Work out the finished part from the listing and answer in its coordinate system (mm). A direction names the side the tool comes from. Round coordinates to 2 decimals unless told otherwise and drop trailing zeros. Loops run counter-clockwise (first coordinate to the right, second up) from the corner with the lowest first, then second, coordinate; pieces in that order, holes last. Notation, with made-up numbers: M -21.5,54.5 L 25.5,54.5 A3 ccw 25.5,59.5 Z; hole C 14.25,80.5 d7. An arc over 180 degrees is marked long. One line per item, written item: value.
Autodesk Inventor part; units mm, degrees
ref_plane "YZ Plane" through (0, 0, 0) normal (1, 0, 0) x (0, 1, 0)
ref_plane "XZ Plane" through (0, 0, 0) normal (0, 1, 0) x (-1, 0, 0)
ref_plane "XY Plane" through (0, 0, 0) normal (0, 0, 1) x (1, 0, 0)
sketch "Sketch1" plane through (0, 0, 0) normal (0, 0, 1) x (1, 0, 0)
  circle A0 centre (0, 24.7) radius 8.1
  line L0 (0, 24.7) -> (0, 0) construction
  line L1 (0, 0) -> (-20, 0) construction
  line L2 (-20, 5) -> (-9.2, 5)
  line L3 (-9.2, 5) -> (-3.85, 17.5735)
  line L4 (0, 0) -> (20, 0) construction
  line L5 (20, 0) -> (20, 5) construction
  line L6 (20, 5) -> (9.2, 5)
  line L7 (9.2, 5) -> (3.85, 17.5735)
  line L8 (0, 24.7) -> (0, 32.8) construction
  line L9 (-3.85, 17.5735) -> (3.85, 17.5735) construction
  line L10 (-20, 5) -> (-20, 42)
  line L11 (-20, 42) -> (20, 42)
  line L12 (20, 42) -> (20, 5)
  line L13 (-20, 5) -> (-20, 0)
  line L14 (-20, 0) -> (20, 0)
  line L15 (20, 0) -> (20, 5)
  line L16 (-9.2, 5) -> (9.2, 5)
  point P0 (0, 42)
  point P1 (-20, 5)
  dimension "d0" = 16.2
  dimension "d2" = 5
  dimension "d5" = 7.7
  dimension "d91" = 42
  dimension "d102" = 19.7
  dimension "d103" = 18.4
  dimension "d104" = 40
extrude "Extrusion1" add sketch "Sketch1" along normal blind 30 contours A0 L3 L2 L10 L11 L12 L6 L7
extrude "Extrusion2" add sketch "Sketch1" against normal blind 10
sketch "Sketch6" plane through (-20, 42, 30) normal (0, 1, 0) x (1, 0, 0)
  line L0 (0, 40) -> (0, 0)
  line L1 (40, 0) -> (0, 0)
  line L2 (0, 40) -> (40, 0) construction
  line L3 (40, 40) -> (0, 0) construction
  circle A0 centre (35, 5) radius 1.5
  circle A1 centre (5, 5) radius 1.5
  circle A2 centre (5, 35) radius 1.5
  circle A3 centre (35, 35) radius 1.5
  line L4 (35, 35) -> (35, 5) construction
  line L5 (5, 5) -> (35, 5) construction
  line L6 (5, 5) -> (5, 35) construction
  circle A4 centre (20, 20) radius 1.5
  line L7 (40, 40) -> (40, 0)
  line L8 (0, 40) -> (40, 40)
  point P0 (20, 30)
  dimension "d69" = 30
  dimension "d70" = 3
  dimension "d73" = 3
extrude "Extrusion8" cut sketch "Sketch6" against normal blind 5 contours A0 | A1 | A2 | A3
extrude "Extrusion9" cut sketch "Sketch6" against normal through all contours A4
sketch "Sketch8" plane through (20, 5, 30) normal (1, 0, 0) x (0, 0, -1)
  line L0 (0, 0) -> (0, 37)
  line L1 (30, 0) -> (0, 0)
  line L2 (20, 37) -> (20, 15) construction
  line L3 (20, 15) -> (10, 15) construction
  line L4 (20, 15) -> (30, 15) construction
  circle A0 centre (10, 15) radius 1.75
  circle A1 centre (30, 15) radius 1.75
  line L5 (40, 37) -> (0, 37)
  line L6 (30, -5) -> (30, 0)
  line L7 (30, -5) -> (40, -5)
  line L8 (40, 37) -> (40, -5)
  line L9 (20, 33.5954) -> (20, 18.5954) construction
  circle A2 centre (20, 33.5954) radius 1.5
  circle A3 centre (20, 18.5954) radius 1.5
  line L10 (20, 26.0954) -> (0, 26.0954) construction
  point P0 (30, -5)
  point P1 (35, -5)
  dimension "d97" = 3.5
  dimension "d98" = 3.5
  dimension "d105" = 20
  dimension "d106" = 20
  dimension "d107" = 20
  dimension "d108" = 15
  dimension "d109" = 20
  dimension "d110" = 3
extrude "Extrusion12" cut sketch "Sketch8" against normal blind 5 contours A0 | A1 | A2 | A3
mirror "Mirror1" about plane through (0, 0, 0) normal (1, 0, 0) of "Extrusion12"
properties part number "X Axis End_3DPrint"
1) The mould has two halves that part along Y. Classify faces 6 (the face through (-17.54, 25.06, 10.33)), 7 (the face through (17.54, 37.68, 11.19)), 8 (the face through (-15, 37, 25)), 9 (the face through (0, 0, -5)): +Y half, -Y half, draft (parallel to the pull), parting line (faces both ways), or undercut.
Check values:
face 6: undercut
face 7: undercut
face 8: +Y half
face 9: -Y half
2) For faces 1 (the face through (-0.3, 32.794, 14.79)), 2 (the face through (-15, 5, 15)), 3 (the face through (15, 24, 10)), 4 (the face through (-6.56, 11.2, 14.79)), 5 (the face through (-17.535, 18.265, 0.228)), determine the directions among +Z, -Z, +X, -X, +Y, -Y from which every point of the face is accessible in a straight line to the end or side of a thin tool.
Check values:
face 1: +Z
face 2: +Z, +X, -X, -Y
face 3: +X
face 4: +Z, -Y
face 5: -X
3) Find section B-B (y = 8.5). Give the vertices of the cut face in (x, z).
Check values:
outline: M -20,-10 L 20,-10 L 20,30 L 7.71,30 L 7.71,0 L -7.71,0 L -7.71,30 L -20,30 Z
4) Each of these flat-tipped pins is pushed along its axis until it touches: pin 1 (4.5 mm diameter, centred on y = 20, z = 0, fed in from -X); pin 2 (2 mm diameter, centred on y = 20, z = 20, fed in from -X); pin 3 (1.5 mm diameter, centred on x = -15.5, z = -5, fed in from +Y); pin 4 (2.5 mm diameter, centred on x = 15, z = 25, fed in from -Y). Where does it stop, or does it pass through?
Check values:
pin 1: x = -20
pin 2: x = -15
pin 3: y = 37
pin 4: y = 5
5) Find section D-D (z = 13). Give the vertices of the cut face in (x, y), then the cut area to 3 significant figures.
Check values:
outline: M -20,5 L -9.2,5 L -3.85,17.57 A8.1 cw long 3.85,17.57 L 9.2,5 L 20,5 L 20,42 L -20,42 Z
area: 1,110 mm2
6) Find section A-A (x = 0). Give the vertices of the cut face in (y, z).
Check values:
outline: M 0,-10 L 42,-10 L 42,8.5 L 32.8,8.5 L 32.8,0 L 0,0 Z; M 32.8,11.5 L 42,11.5 L 42,30 L 32.8,30 Z
7) Find the intervals of material crossed by probe 1 along Y at (x, z) = (-17.6, 10); probe 2 along Z at (x, y) = (-15, 40.45); probe 3 along Y at (x, z) = (18, 20), in increasing order. Write a range as from..to.
Check values:
probe 1: 5..22.1, 25.1..37.1, 40.1..42
probe 2: -10..-6.5, -3.5..23.5, 26.5..30
probe 3: 5..18.25, 21.75..42
8) Find section C-C (x = -7). Give the vertices of the cut face in (y, z).
Check values:
outline: M 0,-10 L 42,-10 L 42,30 L 28.78,30 L 28.78,0 L 20.62,0 L 20.62,30 L 10.17,30 L 10.17,0 L 0,0 Z
